Here's how the part is built. I have some questions about the finished solid (model axes, mm). Face numbers are marked on the shaded views. A direction names the side the tool comes from. Round coordinates to 2 decimals unless told otherwise and drop trailing zeros. Write each loop counter-clockwise with the first axis right and the second up, starting at its lowest first coordinate (ties: lowest second). Pieces come first, ordered by that corner, then holes. Notation, with made-up numbers: (6, 38) - (13, 38) arc R25 cw to (13, 53) - close; hole circle Ø5 at (67.5, 0). An arc over 180 degrees is marked (long way). Return JSON: item names as keys, results as strings. Group by question number.
Autodesk Inventor part; units mm, degrees
ref_plane "YZ Plane" through (0, 0, 0) normal (1, 0, 0) x (0, 1, 0)
ref_plane "XZ Plane" through (0, 0, 0) normal (0, 1, 0) x (-1, 0, 0)
ref_plane "XY Plane" through (0, 0, 0) normal (0, 0, 1) x (1, 0, 0)
sketch "Sketch1" plane through (0, 0, 0) normal (0, 0, 1) x (1, 0, 0)
  line L0 (-83.046, 15.2299) -> (66.954, 15.2299)
  line L1 (66.954, 15.2299) -> (66.954, -4.7701)
  line L2 (66.954, -4.7701) -> (-83.046, -4.7701)
  line L3 (-83.046, -4.7701) -> (-83.046, 15.2299)
  point P0 (0, 0)
  dimension "d0" = 150
  dimension "d1" = 20
extrude "Extrusion1" add sketch "Sketch1" along normal blind 10
sketch "Sketch2" plane through (-83.046, -4.7701, 0) normal (-1, 0, 0) x (0, 0, 1)
  point P0 (0, 4.7701)
sketch "Sketch3" plane through (-83.046, -4.7701, 0) normal (-1, 0, 0) x (0, 0, 1)
  line L0 (0, 20) -> (-4, 20)
  line L1 (-4, 20) -> (-4, 0)
  line L2 (-4, 0) -> (0, 0)
  line L3 (0, 0) -> (0, 20)
  line L4 (10, 0) -> (14, 0)
  line L5 (14, 0) -> (14, 20)
  line L6 (14, 20) -> (10, 20)
  line L7 (10, 20) -> (10, 0)
  line L8 (0, 0) -> (10, 0)
  line L9 (10, 20) -> (10, 0)
  point P0 (0, 4.7701)
  dimension "d4" = 4
  dimension "d5" = 4
extrude "Extrusion2" add sketch "Sketch3" against normal blind 5
sketch "Sketch4" plane through (-83.046, -4.7701, 14) normal (-1, 0, 0) x (0, 0, 1)
  line L0 (-18, 20) -> (-14, 20)
  line L1 (-14, 20) -> (-14, 0)
  line L2 (-14, 0) -> (-18, 0)
  line L3 (-18, 0) -> (-18, 20)
  line L4 (0, 20) -> (-4, 20)
  line L5 (-4, 20) -> (-4, 0)
  line L6 (-4, 0) -> (0, 0)
  line L7 (0, 0) -> (0, 20)
  point P0 (-14, 4.7701)
extrude "Extrusion3" add sketch "Sketch4" along normal blind 30
sketch "Sketch5" plane through (-78.046, -4.7701, 14) normal (0, 0, 1) x (1, 0, 0)
  line L0 (-35, 0) -> (-35, 20)
  line L1 (-5, 20) -> (-35, 20)
  line L2 (-5, 0) -> (-5, 20)
  point P0 (78.046, 4.7701)
  point P1 (-30, 15)
  point P2 (-10, 15)
  dimension "d10" = 5
  dimension "d11" = 5
  dimension "d12" = 5
  dimension "d13" = 5
hole "Hole1" at (-108.046, 10.2299, 14) at (-88.046, 10.2299, 14) direction (0, 0, -1) diameter 3 depth 30 tip angle 118 countersink diameter 6 countersink angle 90
chamfer "Chamfer1" distance 4 angle 45 2 edges at (-78.046, 5.2299, 10) (-78.046, 5.2299, 0)
sketch "Sketch6" plane through (66.954, -4.7701, 0) normal (0, -1, 0) x (1, 0, 0)
  line L0 (0, -4) -> (-5, -4)
  line L1 (-5, -4) -> (-5, 14)
  line L2 (-5, 14) -> (0, 14)
  line L3 (0, 14) -> (0, -4)
  line L4 (0, 0) -> (-141, 0)
  line L5 (-141, 10) -> (0, 10)
  line L6 (0, 0) -> (0, 10)
  point P0 (-66.954, 0)
  dimension "d24" = 4
  dimension "d25" = 4
  dimension "d26" = 5
extrude "Extrusion4" add sketch "Sketch6" against normal blind 20
sketch "Sketch7" plane through (-113.046, -4.7701, 10) normal (0, -1, 0) x (1, 0, 0)
  line L0 (180, -14) -> (210, -14)
  line L1 (210, -14) -> (210, -10)
  line L2 (210, -10) -> (180, -10)
  line L3 (180, -10) -> (180, -14)
  line L4 (180, 4) -> (210, 4)
  line L5 (210, 4) -> (210, 0)
  line L6 (210, 0) -> (180, 0)
  line L7 (180, 0) -> (180, 4)
  point P0 (113.046, -10)
  dimension "d29" = 30
  dimension "d30" = 30
  dimension "d31" = 4
  dimension "d32" = 4
extrude "Extrusion5" add sketch "Sketch7" against normal blind 20
chamfer "Chamfer2" distance 4 angle 45 2 edges at (61.954, 5.2299, 10) (61.954, 5.2299, 0)
sketch "Sketch8" plane through (96.954, -4.7701, 14) normal (0, 0, 1) x (1, 0, 0)
  line L0 (-30, 20) -> (-30, 0)
  line L1 (0, 0) -> (0, 20)
  line L2 (-35, 20) -> (0, 20)
  line L3 (-35, 0) -> (0, 0)
  circle A0 centre (-25, 5) radius 2
  circle A1 centre (-25, 15) radius 2
  circle A2 centre (-5, 5) radius 2
  circle A3 centre (-5, 15) radius 2
  line L4 (-25, 3) -> (-5, 3)
  line L5 (-5, 7) -> (-25, 7)
  line L6 (-25, 13) -> (-5, 13)
  line L7 (-5, 17) -> (-25, 17)
  point P0 (-96.954, 4.7701)
  dimension "d38" = 5
  dimension "d39" = 5
  dimension "d40" = 5
  dimension "d41" = 5
  dimension "d42" = 5
  dimension "d43" = 5
  dimension "d44" = 5
  dimension "d45" = 5
  dimension "d46" = 4
  dimension "d47" = 4
  dimension "d48" = 4
  dimension "d49" = 4
extrude "Extrusion6" cut sketch "Sketch8" against normal blind 20 contours A0 | A0 L5 A2 L4 | A2 | A1 | A1 L7 A3 L6 | A3
sketch "Sketch9" plane through (-113.046, -4.7701, 10) normal (0, -1, 0) x (1, 0, 0)
  line L0 (30, -10) -> (31.8516, -10)
  line L1 (31.8516, -10) -> (31.8516, 0)
  line L2 (31.8516, 0) -> (30, 0)
  line L3 (30, 0) -> (30, -10)
  line L4 (30, 0) -> (0, 0)
  point P0 (113.046, -10)
  dimension "d52" = 1.8516
extrude "Extrusion7" cut sketch "Sketch9" against normal blind 20
sketch "Sketch10" plane through (-113.046, 15.2299, 14) normal (0, 1, 0) x (1, 0, 0)
  line L0 (171, 4) -> (210, 4)
  line L1 (210, 4) -> (210, 0)
  line L2 (210, 0) -> (171, 0)
  line L3 (171, 0) -> (171, 4)
  line L4 (210, 18) -> (171, 18)
  line L5 (171, 18) -> (171, 14)
  line L6 (171, 14) -> (210, 14)
  line L7 (210, 14) -> (210, 18)
  line L8 (180, 14) -> (210, 14)
  point P0 (113.046, 14)
extrude "Extrusion8" cut sketch "Sketch10" against normal blind 20
sketch "Sketch11" plane through (66.954, 15.2299, 10) normal (0, 1, 0) x (1, 0, 0)
  line L0 (0, 0) -> (0, 10)
  line L1 (0, 3.5) -> (20, 3.5)
  line L2 (20, 3.5) -> (20, 6.5)
  line L3 (20, 6.5) -> (0, 6.5)
  line L4 (0, 6.5) -> (0, 3.5)
  line L5 (0, 0) -> (-141, 0)
  point P0 (-66.954, 10)
  dimension "d57" = 3
  dimension "d58" = 3.5
  dimension "d59" = 20
extrude "Extrusion9" add sketch "Sketch11" against normal blind 20
sketch "Sketch12" plane through (66.954, 15.2299, 6.5) normal (0, 0, 1) x (1, 0, 0)
  line L0 (20, -20) -> (0, -20)
  line L1 (20, 0) -> (20, -20)
  point P0 (-66.954, -15.2299)
  point P1 (15, -10)
  dimension "d62" = 10
  dimension "d63" = 5
hole "Hole2" at (81.954, 5.2299, 6.5) direction (0, 0, -1) diameter 3 depth 8 tip angle 118
chamfer "Chamfer3" distance 5 angle 45 2 edges at (86.954, -4.7701, 5) (86.954, 15.2299, 5)
chamfer "Chamfer4" distance 3.5 angle 45 2 edges at (66.954, 5.2299, 6.5) (66.954, 5.2299, 3.5)
properties part number "Upper Support beam v2"
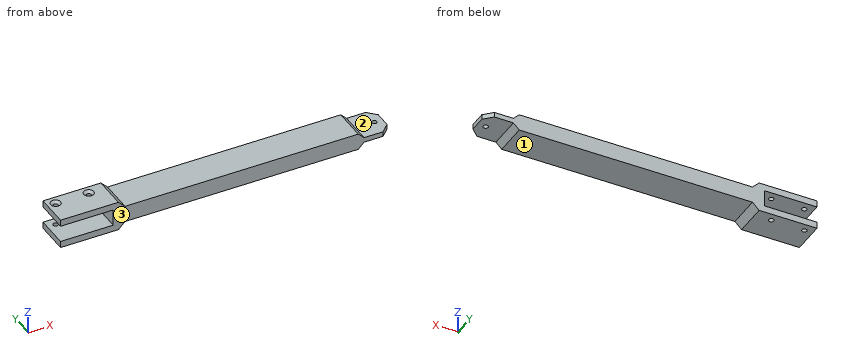
1) Imagine slicing it at B-B (x = 30.5). Please give me the cut outline in (y, z).
2) Imagine slicing it at A-A (x = -97.5). Please give me the cut outline in (y, z), plus the area to 3 significant figures.
3) I need wall thicknesses on line 1 along X through (y, z) = (9.25, -2.75); line 2 along Z through (x, y) = (-85, 11.25); line 3 along Z through (x, y) = (53.5, 7.5). Which ranges of each line are inside material? Lowest first, please.
4) Will these pins go through, and if not, where does the flat tip stop? pin 1 Ø4 at (y, z) = (0.5, 3) entering from -X; pin 2 Ø4 at (x, y) = (-108.05, 10.23) entering from +Z; pin 3 Ø2.5 at (x, y) = (81.95, 5.23) entering from -Z; pin 4 Ø6 at (x, y) = (-14, 6) entering from -Z.
5) For the marked faces 1, 2 and 3, which set-ups out of +Z, -Z, +X, -X, +Y, -Y let a thin tool reach every point of the face, with its end or its side?
Results found:
{
 "1": {"outline": "(-4.77, 0) - (15.23, 0) - (15.23, 10) - (-4.77, 10) - close"},
 "2": {"outline": "(-4.77, -4) - (15.23, -4) - (15.23, 0) - (-4.77, 0) - close; (-4.77, 10) - (15.23, 10) - (15.23, 14) - (-4.77, 14) - close", "area": "160 mm²"},
 "3": {"line 1": "x = -113.05 to -109.18, -106.91 to -89.18, -86.91 to -76.8", "line 2": "z = -4 to 0, 10 to 14", "line 3": "z = 0 to 10"},
 "4": {"pin 1": "stops at x = -81.19", "pin 2": "stops at z = 13", "pin 3": "passes through", "pin 4": "stops at z = 0"},
 "5": {"face 1": "-Z, +X, +Y, -Y", "face 2": "+Z, +X, +Y, -Y", "face 3": "+Z, -Z, +X, -X, -Y"}
}
